```python
from build123d import *

# Parameters (mm, degrees)
SKETCH1_R           = 1.6
BOSS_EXTRUDE1_DEPTH = 5.9944


with BuildPart() as part:
    # Sketch1 → Boss-Extrude1 (new body)
    with BuildSketch(Plane.XY):
        with BuildLine():
            Line((316.995622149, 78.216780382), (326.749772708, 25.13420903))
            ThreePointArc((326.749772708, 25.13420903), (330.912307442, 20.282357802), (337.186376688, 21.508412799))
            Line((337.186376688, 21.508412799), (380.686318009, 59.686636906))
            ThreePointArc((380.686318009, 59.686636906), (381.539726589, 61.358310991), (381.012274461, 63.159586846))
            ThreePointArc((381.012274461, 63.159586846), (381.827165591, 71.841961695), (390.541875435, 71.52335081))
            ThreePointArc((390.541875435, 71.52335081), (392.259481176, 70.76662697), (394.027759373, 71.395906456))
            Line((394.027759373, 71.395906456), (402.058752504, 78.4444))
            Line((402.058752504, 78.4444), (380.453796067, 78.4444))
            Line((380.453796067, 78.4444), (380.453796067, 84.4388))
            Line((380.453796067, 84.4388), (367.753796067, 84.4388))
            Line((367.753796067, 84.4388), (367.753796067, 78.4444))
            Line((367.753796067, 78.4444), (355.053796067, 78.4444))
            Line((355.053796067, 78.4444), (355.053796067, 84.4388))
            Line((355.053796067, 84.4388), (342.353796067, 84.4388))
            Line((342.353796067, 84.4388), (342.353796067, 78.4444))
            Line((342.353796067, 78.4444), (329.653796067, 78.4444))
            Line((329.653796067, 78.4444), (329.653796067, 84.4388))
            Line((329.653796067, 84.4388), (316.953796067, 84.4388))
            Line((316.953796067, 84.4388), (316.953796067, 78.675830573))
            ThreePointArc((316.953796067, 78.675830573), (316.9642742, 78.445354708), (316.995622149, 78.216780382))
        make_face()
        with Locations((332.996689228, 26.282106781)):
            Circle(SKETCH1_R, mode=Mode.SUBTRACT)
        with BuildLine():
            Line((339.346689286, 72.45), (337.033543957, 72.45))
            ThreePointArc((337.033543957, 72.45), (336.440455672, 72.520213312), (335.880156908, 72.726971429))
            ThreePointArc((335.880156908, 72.726971429), (326.660420383, 67.486768409), (335.113137596, 61.08248539))
            ThreePointArc((335.113137596, 61.08248539), (335.530243547, 61.19114772), (335.95971692, 61.227719546))
            Line((335.95971692, 61.227719546), (339.346689286, 61.227719546))
            Line((339.346689286, 61.227719546), (367.753796067, 61.227719546))
            Line((367.753796067, 61.227719546), (367.753796067, 72.45))
            Line((367.753796067, 72.45), (339.346689286, 72.45))
        make_face(mode=Mode.SUBTRACT)
    extrude(amount=BOSS_EXTRUDE1_DEPTH)


solid = part.part
```
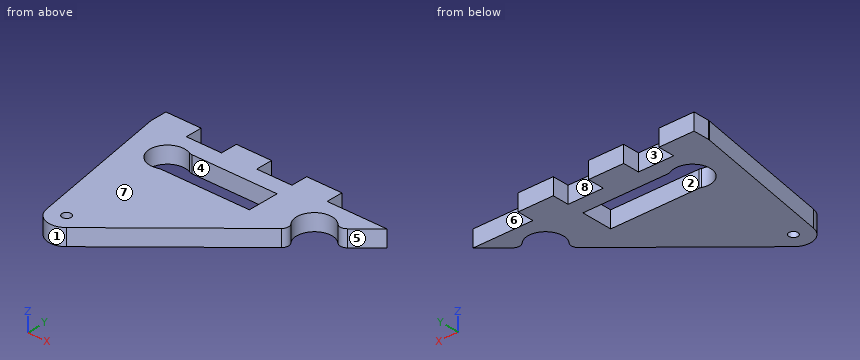
Here's how the part is built. I have some questions about the finished solid (model axes, mm). Face numbers are marked on the shaded views. A direction names the side the tool comes from. Give positions to 0.01 mm unless a question says otherwise; leave off trailing zeros. Loops run counter-clockwise (first coordinate to the right, second up) from the corner with the lowest first, then second, coordinate; pieces in that order, holes last. Notation, with made-up numbers: M 48.25,71.25 L 86.25,71.25 A24 ccw 86.25,91.25 Z; hole C -16,-29 d9. An arc over 180 degrees is marked long. Return JSON: item names as keys, results as strings.
Item 1: Imagine slicing it at C-C on z = 4. List the corners of the cut face in (x, y) for me, then the cut area to 3 significant figures.
A:
{"outline": "M 316.95,78.68 A2.54 ccw 317,78.22 L 326.75,25.13 A6.35 ccw 337.19,21.51 L 380.69,59.69 A2.54 ccw 381.01,63.16 A6.35 cw 390.54,71.52 A2.54 ccw 394.03,71.4 L 402.06,78.44 L 380.45,78.44 L 380.45,84.44 L 367.75,84.44 L 367.75,78.44 L 355.05,78.44 L 355.05,84.44 L 342.35,84.44 L 342.35,78.44 L 329.65,78.44 L 329.65,84.44 L 316.95,84.44 Z; hole C 333,26.28 d3.2; hole M 335.11,61.08 A2.54 cw 335.96,61.23 L 367.75,61.23 L 367.75,72.45 L 337.03,72.45 A2.54 cw 335.88,72.73 A6.35 ccw long Z", "area": "2,380 mm^2"}
Item 2: Imagine slicing it at B-B on y = 65.5. List the corners of the cut face in (x, z) for me.
A:
{"outline": "M 319.33,0 L 326.84,0 L 326.84,5.99 L 319.33,5.99 Z; M 367.75,0 L 379.86,0 L 379.86,5.99 L 367.75,5.99 Z"}
Item 3: Imagine slicing it at A-A on x = 361. List the corners of the cut face in (y, z) for me.
A:
{"outline": "M 42.41,0 L 61.23,0 L 61.23,5.99 L 42.41,5.99 Z; M 72.45,0 L 78.44,0 L 78.44,5.99 L 72.45,5.99 Z"}
Item 4: Please list where these lines run through material, in increasing order: line 1 (Y direction, x = 362, z = 2.95); line 2 (Y direction, x = 386, z = 2.3); line 3 (X direction, y = 70.5, z = 1.65).
A:
{"line 1": "y = 43.29 to 61.23, 72.45 to 78.44", "line 2": "y = 73.42 to 78.44", "line 3": "x = 318.41 to 327.65, 367.75 to 380.67"}
Item 5: I'm going to push flat-ended pins straight in: pin 1 Ø1.8 at (y, z) = (82, 4) entering from +X; pin 2 Ø1.5 at (y, z) = (62.5, 1) entering from +X; pin 3 Ø2 at (y, z) = (68.5, 1) entering from +X; pin 4 Ø7.5 at (x, y) = (333, 67.07) entering from -Z. Where does each tip first touch, or does it pass through?
A:
{"pin 1": "stops at x = 380.45", "pin 2": "stops at x = 381.55", "pin 3": "stops at x = 380.15", "pin 4": "passes through"}
Item 6: Imagine slicing it at D-D on y = 41.5. List the corners of the cut face in (x, z) for me, then the cut area to 3 significant figures.
A:
{"outline": "M 323.74,0 L 359.96,0 L 359.96,5.99 L 323.74,5.99 Z", "area": "217 mm^2"}
Item 7: Thinking about a two-plate mould opening in Y: for the marked faces 1, 2 and 3, which applies, released by +Y, released by -Y, zero draft, split by the parting line, or undercut?
A:
{"face 1": "released by -Y", "face 2": "undercut", "face 3": "released by +Y"}
Item 8: On a 3-axis mill with a long thin cutter (end or side, diameter ignored), from which of +Z, -Z, +X, -X, +Y, -Y can I reach the whole of each face in a straight line? I mean the marked faces 4, 5, 6, 7 and 8. Say none if no direction works.
A:
{"face 4": "+Z, -Z", "face 5": "+Z, -Z, +X, -Y", "face 6": "+Z, -Z, +X, +Y", "face 7": "+Z, +X, -X, +Y, -Y", "face 8": "+Z, -Z, +Y"}
